Verification items for the finished model (mm, model axes). Face numbers are marked on the shaded views. A direction names the side the tool comes from. Round coordinates to 2 decimals unless told otherwise and drop trailing zeros. Loops run counter-clockwise (first coordinate to the right, second up) from the corner with the lowest first, then second, coordinate; pieces in that order, holes last.
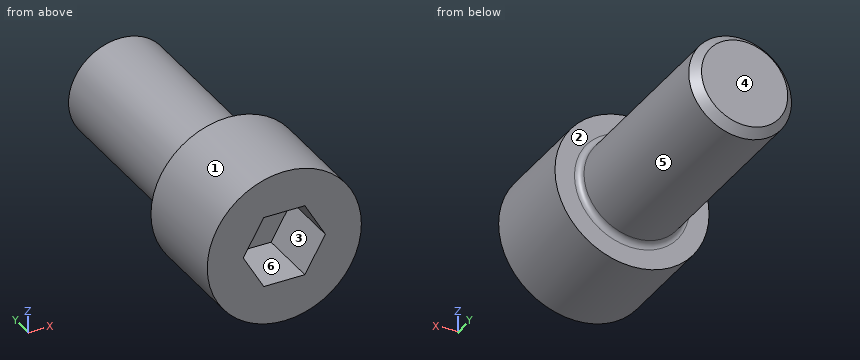
from build123d import *

# Parameters (mm, degrees)
SKETCH2_R           = 4.7625
BOSS_EXTRUDE1_DEPTH = 6.35
CUT_EXTRUDE1_DEPTH  = 3.81
SKETCH4_R           = 3.175
BOSS_EXTRUDE5_DEPTH = 12.7
FILLET2_R           = 0.381
CHAMFER1_SIZE       = 0.508


with BuildPart() as part:
    # Sketch2 → Boss-Extrude1 (new body)
    with BuildSketch(Plane(origin=(0, 0, 0), x_dir=(1, 0, 0), z_dir=(0, 1, 0))):
        Circle(SKETCH2_R)
    extrude(amount=BOSS_EXTRUDE1_DEPTH)

    # Sketch3 → Cut-Extrude1 (cut)
    with BuildSketch(Plane.XZ):
        Polygon((2.54, 0), (1.27, 2.199704526), (-1.27, 2.199704526), (-2.54, 0), (-1.27, -2.199704526), (1.27, -2.199704526), align=None)
    extrude(amount=-CUT_EXTRUDE1_DEPTH, mode=Mode.SUBTRACT)

    # Sketch4 → Boss-Extrude5 (add)
    with BuildSketch(Plane(origin=(0, 6.35, 0), x_dir=(1, 0, 0), z_dir=(0, 1, 0))):
        Circle(SKETCH4_R)
    extrude(amount=BOSS_EXTRUDE5_DEPTH)

    # Fillet2
    fillet2_edges = [part.edges().sort_by_distance(p)[0] for p in [
        (-3.175, 6.35, 0),
    ]]
    fillet(fillet2_edges, radius=FILLET2_R)

    # Chamfer1
    chamfer1_edges = [part.edges().sort_by_distance(p)[0] for p in [
        (-3.175, 19.05, 0),
    ]]
    chamfer(chamfer1_edges, length=CHAMFER1_SIZE)


solid = part.part
1. Tool access check on the marked faces 4, 5 and 6. Record the directions out of +Z, -Z, +X, -X, +Y, -Y that give a thin tool (end or side, any length) a straight path to the whole face; none if there is none.
2. Release check for a two-part mould opening along Z. For the marked faces 1, 2 and 3 record: released by +Z, released by -Z, zero draft, split by the parting line, or undercut.
3. Section check B-B (y = 4). Enter the section's corners in (x, z) (1 decimal), then the cut area to 3 significant figures.
4. Gauge pin test, flat ends, axial feed: P1, Ø3, axis at x = -0.5, y = 1, coming from the -Z side; P2, Ø3, axis at y = 16, z = -1, coming from the +X side (3 decimals); P3, Ø4, axis at x = -3.5, y = 15, coming from the -Z side; P4, Ø5, axis at y = 9, z = -3, coming from the -X side. Record the tip position at first contact, or that the pin passes through.
5. Scan lines: L1, parallel to Y at x = 1.75, z = 1; L2, parallel to X at y = 7, z = 0 (3 decimals); L3, parallel to Y at x = 2.25, z = 2.75. Record each from-to range of solid material in increasing order.
6. Section check C-C (y = 17). Enter the section's corners in (x, z) (3 decimals).
7. Section check D-D (x = 3.75). Enter the section's corners in (y, z), then the cut area to 3 significant figures.
Taken from the geometry:
1. face 4: +Z, -Z, +X, -X, +Y
1. face 5: +Y
1. face 6: -Y
2. face 1: split by the parting line
2. face 2: zero draft
2. face 3: undercut
3. outline: circle Ø9.5 at (0, 0)
3. area: 71.3 mm2
4. P1: stops at z = -4.76
4. P2: stops at x = 3.175
4. P3: stops at z = -2.8
4. P4: stops at x = -3.14
5. L1: y = 3.81 to 19.05
5. L2: x = -3.175 to 3.175
5. L3: y = 0 to 6.35
6. outline: circle Ø6.35 at (0, 0)
7. outline: (0, -2.94) - (6.35, -2.94) - (6.35, 2.94) - (0, 2.94) - close
7. area: 37.3 mm2
